Input: dimensioned drawing with shaded views. Units: mm. Origin: part minimum x, y, z. A direction names the side the tool comes from. Coordinates: 2 decimals unless noted, no trailing zeros. Order: outer loops, then holes, each group sorted by start corner. A loop starts at its lowest first (then second) coordinate and runs counter-clockwise, first axis right, second up. Notation, with made-up numbers: (65, 61.5) -> (124, 61.5) arc R13 cw to (124, 80.5) -> close; hole circle Ø2 at (12.5, 52). An arc over 180 degrees is marked (long way). Answer in a Markdown table with one row per item. Add a question column.
1) Section query D-D on z = 2.8. Return the cut outline in (x, y) (1 decimal).
2) Contact query for flat-ended pins moving along their axis: P1, Ø1.6, axis at x = 5.5, y = 12, coming from the +Z side (1 decimal); P2, Ø1.5, axis at y = 12.5, z = 1.5, coming from the -X side. Output: stop coordinate, or through.
3) Section query C-C on y = 7.5. Return the cut outline in (x, z) (1 decimal).
4) Section query B-B on x = 5.08. Return the cut outline in (y, z) (1 decimal).
5) Ray query, line 1 (X direction, y = 13.25, z = 1.8); line 2 (Z direction, x = 3.75, y = 12.25) (1 decimal); line 3 (X direction, y = 5.75, z = 2.95) (1 decimal). Return the intervals inside material, ascending. Write a range as from..to.
6) Section query A-A on z = 0.6. Return the cut outline in (x, y) (1 decimal).
7) Set-up query: the marked faces 1, 2 and 3. Return all of +Z, -Z, +X, -X, +Y, -Y with unobstructed straight access to the full face (end or side cutting, diameter ignored); none if empty.
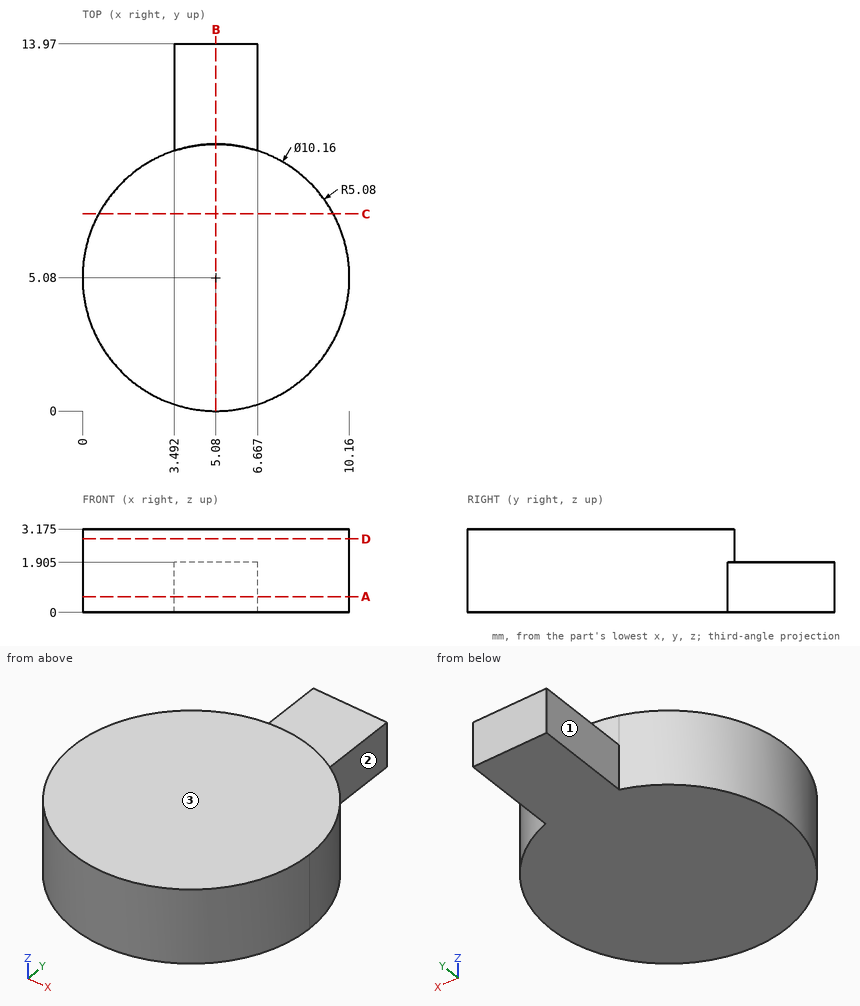
Result:
| question | item | result |
|---|---|---|
| 1 | outline | (3.5, 9.9) arc R5.1 ccw (long way) to (6.7, 9.9) arc R5.1 ccw to start |
| 2 | P1 | z = 1.9 |
| 2 | P2 | x = 3.49 |
| 3 | outline | (0.6, 0) -> (9.5, 0) -> (9.5, 3.2) -> (0.6, 3.2) -> close |
| 4 | outline | (0, 0) -> (14, 0) -> (14, 1.9) -> (10.2, 1.9) -> (10.2, 3.2) -> (0, 3.2) -> close |
| 5 | line 1 | 3.49..6.67 |
| 5 | line 2 | 0..1.9 |
| 5 | line 3 | 0..10.1 |
| 6 | outline | (3.5, 9.9) arc R5.1 ccw (long way) to (6.7, 9.9) -> (6.7, 14) -> (3.5, 14) -> close |
| 7 | face 1 | +Z, -Z, -X, +Y |
| 7 | face 2 | +Z, -Z, +X, +Y |
| 7 | face 3 | +Z, +X, -X, +Y, -Y |
